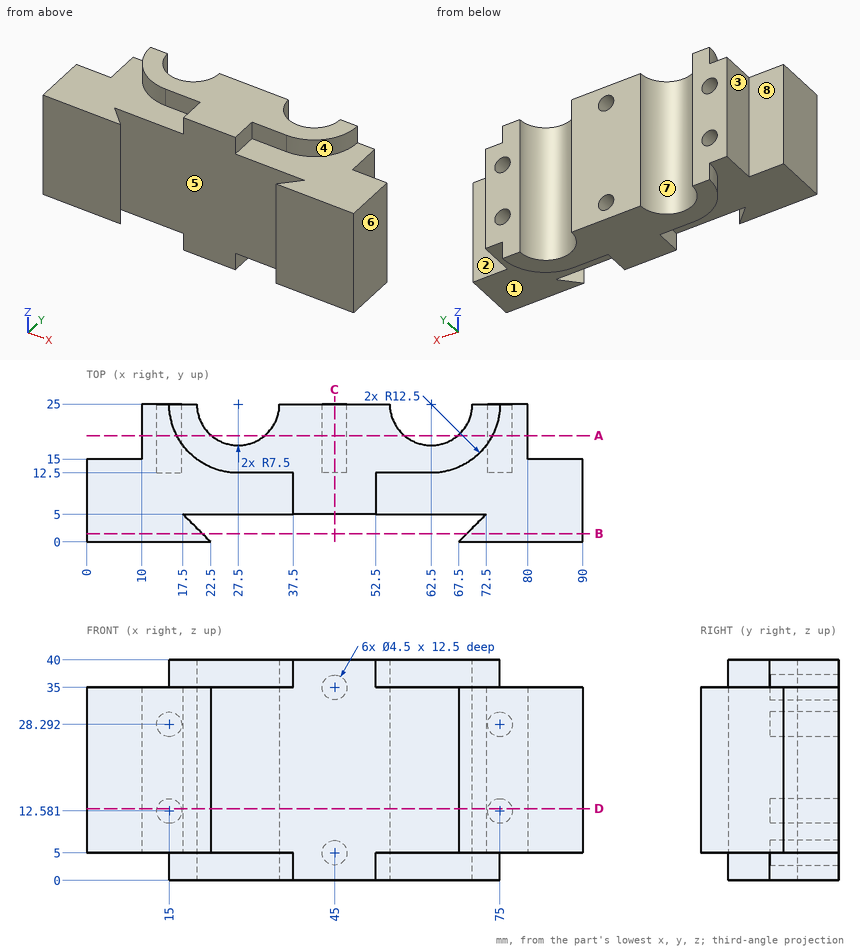
Print and shaded views of the part. All mm, measured from the part's lowest x, y and z. A direction names the side the tool comes from. Coordinates: 2 decimals unless noted, no trailing zeros. Order: outer loops, then holes, each group sorted by start corner. A loop starts at its lowest first (then second) coordinate and runs counter-clockwise, first axis right, second up.
Item 1: Saw through at C-C on x = 45. List the corners of the cut face in (y, z).
Filled in:
outline: (5, 0) - (25, 0) - (25, 2.75) - (12.5, 2.75) - (12.5, 7.25) - (25, 7.25) - (25, 32.75) - (12.5, 32.75) - (12.5, 37.25) - (25, 37.25) - (25, 40) - (5, 40) - close
Item 2: Tool access for the marked faces 1, 2, 3 and 4: list every direction of +Z, -Z, +X, -X, +Y, -Y with a clear straight run to the whole face (end or side of a thin tool).
Filled in:
face 1: -Z, +X, -Y
face 2: +Z, -Z, +X, +Y
face 3: +Z, -Z, -X, +Y
face 4: +Z, +X, -Y
Item 3: Drill centre lines: L1, parallel to Z at x = 75, y = 15.75; L2, parallel to X at y = 23, z = 24; L3, parallel to X at y = 19, z = 22.5. Where is each one in solid material? Low to high.
Filled in:
L1: z = 5 to 10.33, 14.83 to 26.04, 30.54 to 35
L2: x = 10 to 20.27, 34.73 to 55.27, 69.73 to 80
L3: x = 10 to 23, 32 to 58, 67 to 80
Item 4: Saw through at B-B on y = 1.5. List the corners of the cut face in (x, z).
Filled in:
outline: (0, 5) - (21, 5) - (21, 35) - (0, 35) - close; (69, 5) - (90, 5) - (90, 35) - (69, 35) - close
Item 5: Mould opens along X. For the marked faces 5, 6, 7 and 8 say: released by +X, released by -X, zero draft, split by the parting line, or undercut.
Filled in:
face 5: undercut
face 6: released by +X
face 7: undercut
face 8: zero draft
Item 6: Saw through at D-D on z = 13. List the corners of the cut face in (x, y), then the cut area to 3 significant figures.
Filled in:
outline: (0, 0) - (22.5, 0) - (17.5, 5) - (72.5, 5) - (67.5, 0) - (90, 0) - (90, 15) - (80, 15) - (80, 25) - (77.21, 25) - (77.21, 12.5) - (72.79, 12.5) - (72.79, 25) - (70, 25) arc R7.5 cw to (55, 25) - (35, 25) arc R7.5 cw to (20, 25) - (17.21, 25) - (17.21, 12.5) - (12.79, 12.5) - (12.79, 25) - (10, 25) - (10, 15) - (0, 15) - close
area: 1,510 mm2
Item 7: Saw through at A-A on y = 19.25. State how many separate pieces and enclosed holes the cut face has, then the cut area to 3 significant figures.
Filled in:
separate pieces: 3
enclosed holes: 6
area: 1,810 mm2
Item 8: Drop flat-ended pins along their axis: pin 1 Ø5 at (x, z) = (84.5, 16.5) entering from +Y; pin 2 Ø2.5 at (x, z) = (59.5, 2) entering from -Y; pin 3 Ø3 at (y, z) = (20.5, 14) entering from -X. Give the stop position or say it passes through.
Filled in:
pin 1: stops at y = 15
pin 2: stops at y = 12.5
pin 3: stops at x = 10
